```python
from build123d import *

# Parameters (mm, degrees)
SKETCH1_W           = 18
SKETCH1_H           = 20
BOSS_EXTRUDE1_DEPTH = 1
SKETCH2_W           = 18
SKETCH2_H           = 3
BOSS_EXTRUDE2_DEPTH = 2
SKETCH3_R           = 1.6
CUT_EXTRUDE1_DEPTH  = 27.981475126


with BuildPart() as part:
    # Sketch1 → Boss-Extrude1 (new body)
    with BuildSketch(Plane(origin=(0, 0, 0), x_dir=(1, 0, 0), z_dir=(0, 1, 0))):
        with Locations((9, 10)):
            Rectangle(SKETCH1_W, SKETCH1_H)
    extrude(amount=BOSS_EXTRUDE1_DEPTH)

    # Sketch2 → Boss-Extrude2 (add)
    with BuildSketch(Plane.XY):
        with Locations((9, 0.5)):
            Rectangle(SKETCH2_W, SKETCH2_H)
    extrude(amount=BOSS_EXTRUDE2_DEPTH)

    # Sketch3 → Cut-Extrude1 (cut, through all)
    with BuildSketch(Plane(origin=(0, 1, 0), x_dir=(1, 0, 0), z_dir=(0, 1, 0))):
        with Locations(Location((9, 10, 0), (0, 0, 270))):
            Circle(SKETCH3_R)
    extrude(amount=-CUT_EXTRUDE1_DEPTH, mode=Mode.SUBTRACT)


solid = part.part
```
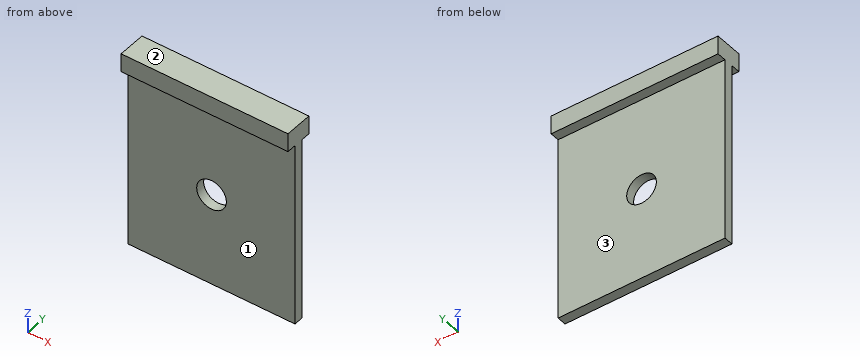
Build history of the part. All positions in model axes, mm. Face numbers are marked on the shaded views. A direction names the side the tool comes from. Give positions to 0.01 mm unless a question says otherwise; leave off trailing zeros. Loops run counter-clockwise (first coordinate to the right, second up) from the corner with the lowest first, then second, coordinate; pieces in that order, holes last.
Item 1: Drill centre lines: line 1 (X direction, y = 0.75, z = -10); line 2 (Z direction, x = 4.25, y = 1.5); line 3 (Y direction, x = 8.75, z = -18.25). Where is each one in solid material? Low to high.
Answers follow:
line 1: x = 0 to 7.4, 10.6 to 18
line 2: z = 0 to 2
line 3: y = 0 to 1
Item 2: Which spindle directions (+Z, -Z, +X, -X, +Y, -Y) get a long thin tool onto all of the face, cutting with end or side? Do the marked faces 1, 2 and 3. Say none if no direction does.
Answers follow:
face 1: -Z, +X, -X, -Y
face 2: +Z, +X, -X, +Y, -Y
face 3: -Z, +X, -X, +Y
Item 3: Slice it at A-A, the plane x = 9. List the corners of the cut face in (y, z).
Answers follow:
outline: (-1, 0) - (0, 0) - (0, -8.4) - (1, -8.4) - (1, 0) - (2, 0) - (2, 2) - (-1, 2) - close; (0, -20) - (1, -20) - (1, -11.6) - (0, -11.6) - close
Item 4: Flat gauge pins, fed straight in: pin 1 (6 mm diameter, centred on x = 15, z = -13, fed in from -Y); pin 2 (4 mm diameter, centred on x = 15, z = -15, fed in from +Y). Where does each tip first touch, or does it go through?
Answers follow:
pin 1: stops at y = 0
pin 2: stops at y = 1
Item 5: Slice it at D-D, the plane x = 5.25. List the corners of the cut face in (y, z).
Answers follow:
outline: (-1, 0) - (0, 0) - (0, -20) - (1, -20) - (1, 0) - (2, 0) - (2, 2) - (-1, 2) - close
Item 6: Slice it at B-B, the plane z = -10. List the corners of the cut face in (x, y), and give its area (3 significant figures).
Answers follow:
outline: (0, 0) - (7.4, 0) - (7.4, 1) - (0, 1) - close; (10.6, 0) - (18, 0) - (18, 1) - (10.6, 1) - close
area: 14.8 mm2
Item 7: Slice it at C-C, the plane y = 0.3. List the corners of the cut face in (x, z), and give its area (3 significant figures).
Answers follow:
outline: (0, -20) - (18, -20) - (18, 2) - (0, 2) - close; hole circle Ø3.2 at (9, -10)
area: 388 mm2
